from build123d import *

# Parameters (mm, degrees)
SKETCH1_W                          = 55.2
SKETCH1_H                          = 30
SKETCH2_W                          = 90
SKETCH2_H                          = 90
BOSS_EXTRUDE1_DEPTH                = 30
SKETCH8_W                          = 96.2
SKETCH8_H                          = 30
SKETCH11_W                         = 100.2
SKETCH11_H                         = 27
SKETCH15_W                         = 2.5
SKETCH15_H                         = 30
SKETCH16_W                         = 20
SKETCH16_H                         = 71.644187242
CUT_EXTRUDE1_DEPTH                 = 55.2
SKETCH17_OUTSIDE_W                 = 124.71
SKETCH17_OUTSIDE_H                 = 124.71
SKETCH17_OUTSIDE_W_2               = 50
SKETCH17_OUTSIDE_H_2               = 73.870600334
CUT_EXTRUDE2_DEPTH                 = 55.2
SKETCH19_R                         = 10
CUT_EXTRUDE3_DEPTH                 = 133.182790105
CUT_EXTRUDE4_DEPTH                 = 133.182790105
TAP_DRILL_FOR_M1_2X0_25_TAP2_D     = 48
TAP_DRILL_FOR_M1_2X0_25_TAP2_DEPTH = 25
TAP_DRILL_FOR_M1_2X0_25_TAP2_TIP   = 14.420654857
CIRPATTERN1_COUNT                  = 4
M16X1_5_TAPPED_HOLE3_D             = 14.5
M16X1_5_TAPPED_HOLE3_DEPTH         = 16
M16X1_5_TAPPED_HOLE3_TIP           = 4.356239488
CUT_EXTRUDE5_REACH                 = 145.779
SKETCH45_R                         = 1.7


with BuildPart() as part:
    # Sketch1 → Revolve-Thin1 (revolve)
    with BuildSketch(Plane.XY, mode=Mode.PRIVATE) as revolve_thin1_sk:
        with Locations((27.6, 15)):
            Rectangle(SKETCH1_W, SKETCH1_H)
    revolve(revolve_thin1_sk.sketch.rotate(Axis((0, 0, 0), (1, 0, 0)), 90), axis=Axis((0, 0, 0), (1, 0, 0)))

    # Sketch2 → Boss-Extrude1 (add)
    with BuildSketch(Plane(origin=(55.2, 0, 0), x_dir=(0, 0, -1), z_dir=(1, 0, 0))):
        Rectangle(SKETCH2_W, SKETCH2_H)
    extrude(amount=BOSS_EXTRUDE1_DEPTH)

    # Sketch8 → Revolve-Thin2 (revolve)
    with BuildSketch(Plane.XY, mode=Mode.PRIVATE) as revolve_thin2_sk:
        with Locations((48.1, 15)):
            Rectangle(SKETCH8_W, SKETCH8_H)
    revolve(revolve_thin2_sk.sketch.rotate(Axis((0, 0, 0), (1, 0, 0)), 90), axis=Axis((0, 0, 0), (1, 0, 0)))

    # Sketch11 → Revolve-Thin3 (revolve)
    with BuildSketch(Plane(origin=(0, 0, 0), x_dir=(1, 0, 0), z_dir=(0, 1, 0)), mode=Mode.PRIVATE) as revolve_thin3_sk:
        with Locations((50.1, 13.5)):
            Rectangle(SKETCH11_W, SKETCH11_H)
    revolve(revolve_thin3_sk.sketch.rotate(Axis((0, 0, 0), (1, 0, 0)), 180), axis=Axis((0, 0, 0), (1, 0, 0)))

    # Sketch15 → Revolve-Thin4 (revolve)
    with BuildSketch(Plane.XY, mode=Mode.PRIVATE) as revolve_thin4_sk:
        with Locations((101.45, 15)):
            Rectangle(SKETCH15_W, SKETCH15_H)
    revolve(revolve_thin4_sk.sketch.rotate(Axis((100.2, 0, 0), (1, 0, 0)), 90), axis=Axis((100.2, 0, 0), (1, 0, 0)))

    # Sketch16 → Cut-Extrude1 (cut)
    with BuildSketch(Plane.ZY):
        Rectangle(SKETCH16_W, SKETCH16_H)
    extrude(amount=-CUT_EXTRUDE1_DEPTH, mode=Mode.SUBTRACT)

    # Sketch17 outside → Cut-Extrude2 (cut)
    with BuildSketch(Plane.ZY):
        Rectangle(SKETCH17_OUTSIDE_W, SKETCH17_OUTSIDE_H)
        Rectangle(SKETCH17_OUTSIDE_W_2, SKETCH17_OUTSIDE_H_2, mode=Mode.SUBTRACT)
    extrude(amount=-CUT_EXTRUDE2_DEPTH, mode=Mode.SUBTRACT)

    # Sketch19 → Cut-Extrude3 (cut, through all)
    with BuildSketch(Plane.XY.offset(25)):
        with Locations((25.2, 0)):
            Circle(SKETCH19_R)
    extrude(amount=-CUT_EXTRUDE3_DEPTH, mode=Mode.SUBTRACT)

    # Sketch22 → Cut-Extrude4 (cut, through all)
    with BuildSketch(Plane(origin=(0, 0, -25), x_dir=(-1, 0, 0), z_dir=(0, 0, -1))):
        with BuildLine():
            Line((0, 16.583123952), (-5, 16.583123952))
            ThreePointArc((-5, 16.583123952), (-1.277186767, 8.660254038), (0, 0))
            Line((0, 0), (0, 16.583123952))
        make_face()
        with BuildLine():
            Line((9.98487255, 34.360502565), (-23.649851102, 34.360502565))
            Line((-23.649851102, 34.360502565), (-23.649851102, 29.320225254))
            ThreePointArc((-23.649851102, 29.320225254), (-13.080591134, 24.773647362), (-5, 16.583123952))
            Line((-5, 16.583123952), (0, 16.583123952))
            Line((0, 16.583123952), (0, 0))
            Line((0, 0), (0, -16.583123952))
            Line((0, -16.583123952), (-5, -16.583123952))
            ThreePointArc((-5, -16.583123952), (-13.080591134, -24.773647362), (-23.649851102, -29.320225254))
            Line((-23.649851102, -29.320225254), (-23.649851102, -35.668103598))
            Line((-23.649851102, -35.668103598), (9.98487255, -35.668103598))
            Line((9.98487255, -35.668103598), (9.98487255, 34.360502565))
        make_face()
        with BuildLine():
            Line((0, -16.583123952), (0, 0))
            ThreePointArc((0, 0), (-1.277186767, -8.660254038), (-5, -16.583123952))
            Line((-5, -16.583123952), (0, -16.583123952))
        make_face()
    extrude(amount=-CUT_EXTRUDE4_DEPTH, mode=Mode.SUBTRACT)

    # Tap Drill for M1.2x0.25 Tap2
    with Locations(Plane(origin=(102.7, 0, 0), x_dir=(0, 0, -1), z_dir=(1, 0, 0))):
        with Locations((0, 0)):
            Hole(TAP_DRILL_FOR_M1_2X0_25_TAP2_D / 2, depth=TAP_DRILL_FOR_M1_2X0_25_TAP2_DEPTH)
            with Locations((0, 0, -(TAP_DRILL_FOR_M1_2X0_25_TAP2_DEPTH + TAP_DRILL_FOR_M1_2X0_25_TAP2_TIP / 2))):  # 118° drill point
                Cone(0, TAP_DRILL_FOR_M1_2X0_25_TAP2_D / 2, TAP_DRILL_FOR_M1_2X0_25_TAP2_TIP, mode=Mode.SUBTRACT)

    # Sketch32 → M12 Tapped Hole2 (revolve, cut)
    with BuildSketch(Plane(origin=(85.2, -31.819805153, 31.819805153), x_dir=(0, 0, -1), z_dir=(0, 1, 0))):
        Polygon((0, 0), (0, 23.064389157), (5.1, 20), (5.1, 0), align=None)
    m12_tapped_hole2 = revolve(axis=Axis((91.55, -31.819805153, 31.819805153), (-1, 0, 0)), mode=Mode.SUBTRACT)

    # CirPattern1: M12 Tapped Hole2 ×4 about axis
    cirpattern1_axis = Axis((0, 0, 0), (1, 0, 0))
    for i in range(1, CIRPATTERN1_COUNT):
        add(m12_tapped_hole2.rotate(cirpattern1_axis, i * 360 / CIRPATTERN1_COUNT), mode=Mode.SUBTRACT)

    # M16x1.5 Tapped Hole3
    with Locations(Plane(origin=(70.2, -45, 0), x_dir=(0, 0, -1), z_dir=(0, -1, 0))):
        with Locations((0, 0)):
            Hole(M16X1_5_TAPPED_HOLE3_D / 2, depth=M16X1_5_TAPPED_HOLE3_DEPTH)
            with Locations((0, 0, -(M16X1_5_TAPPED_HOLE3_DEPTH + M16X1_5_TAPPED_HOLE3_TIP / 2))):  # 118° drill point
                Cone(0, M16X1_5_TAPPED_HOLE3_D / 2, M16X1_5_TAPPED_HOLE3_TIP, mode=Mode.SUBTRACT)

    # Cut-Extrude5: up to this cone (the profile starts outside it)
    cut_extrude5_end = Plane(origin=(70.2, 0, 0), z_dir=(1, 0, 0)).offset(-6.920653857) * Cone(1.664e-06, 274.136053392, 164.717557739, align=(Align.CENTER, Align.CENTER, Align.MIN), mode=Mode.PRIVATE)
    # Sketch45 → Cut-Extrude5 (cut, up to the surface)
    with BuildSketch(Plane.XZ.offset(45), mode=Mode.PRIVATE) as cut_extrude5_sk1:
        with Locations(Location((70.2, 0, 0), (0, 0, 270))):
            Circle(SKETCH45_R)
    cut_extrude5_tool1 = extrude(cut_extrude5_sk1.sketch, amount=-CUT_EXTRUDE5_REACH, mode=Mode.PRIVATE) - cut_extrude5_end
    add(cut_extrude5_tool1.solids().sort_by_distance((70.2, -45, 0))[0], mode=Mode.SUBTRACT)


solid = part.part
Read the model definition and answer for the solid it produces. Units are mm, in the model's axes. A direction names the side the tool comes from. Give positions to 0.01 mm unless a question says otherwise; leave off trailing zeros. Loops run counter-clockwise (first coordinate to the right, second up) from the corner with the lowest first, then second, coordinate; pieces in that order, holes last. Notation, with made-up numbers: (45, 64.5) - (86, 64.5) arc R29 cw to (86, 96.5) - close; hole circle Ø8 at (-7, 64.5). An arc over 180 degrees is marked (long way). Answer as CSV lines item,"result". Start each with the question number.
1) Find section B-B (x = 93). Write down the section's boundary in (y, z), then the cut area to 3 significant figures.
2) Determine the mould class of faces 1 (the face through (62.67, 31.03, -31.41)), 2 (the face through (75.34, -29.866, 27.109)), 3 (the face through (98.23, 26.36, -5.85)) for opening direction X: released by +X, released by -X, zero draft, split by the parting line, or undercut.
3) Which of the six approach directions +Z, -Z, +X, -X, +Y, -Y give full straight-line access (tool end or side, diameter ignored) to faces 4 (the face through (101.468, -25.296, 16.128)), 5 (the face through (33, -7, -10)), 6 (the face through (100.2, -11, 25)), 7 (the face through (36, 24, 18))?
4) Find section C-C (x = 70.2). Write down the section's boundary in (y, z).
5) Straight lines are drawn through the part: L1, parallel to Z at x = 14.5, y = -10; L2, parallel to Z at x = 17, y = -18; L3, parallel to Y at x = 77, z = 35. For each, find the intervals that lie inside material, in ascending order. Write a range as from..to.
6) Each of these flat-tipped pins is pushed along its axis until it touches: pin 1 Ø16 at (x, y) = (25.2, 0) entering from -Z; pin 2 Ø8 at (y, z) = (31.82, -31.82) entering from +X; pin 3 Ø6 at (y, z) = (-31.82, 31.82) entering from +X; pin 4 Ø1 at (y, z) = (26.5, -35.5) entering from +X. Where does it stop, or does it pass through?
7) Find section A-A (x = 46). Write down the section's boundary in (y, z), then the cut area to 3 significant figures.
Findings below:
1,outline,"circle Ø60 at (0, 0); hole circle Ø48 at (0, 0)"
1,area,"1,020 mm^2"
2,face 1,"released by +X"
2,face 2,"zero draft"
2,face 3,"undercut"
3,face 4,"+X"
3,face 5,"-X, +Y, -Y"
3,face 6,"none"
3,face 7,"+Z, -X, +Y"
4,outline,"(-45, -45) - (45, -45) - (45, 45) - (-45, 45) - (-45, 7.25) - (-29, 7.25) - (-25.67, 1.7) - (-11.39, 1.7) arc R11.52 cw (long way) to (-11.39, -1.7) - (-25.67, -1.7) - (-29, -7.25) - (-45, -7.25) - close; hole circle Ø10.2 at (-31.82, -31.82); hole circle Ø10.2 at (-31.82, 31.82); hole circle Ø10.2 at (31.82, -31.82); hole circle Ø10.2 at (31.82, 31.82)"
5,L1,"-25..-10, 10..25"
5,L2,"-24..-10, 10..24"
5,L3,"-45..-35.81, -27.83..27.83, 35.81..45"
6,pin 1,"through"
6,pin 2,"x = 64.54"
6,pin 3,"x = 63.94"
6,pin 4,"x = 85.2"
7,outline,"(-28.28, -10) arc R30 ccw to (-16.58, -25) - (16.58, -25) arc R30 ccw to (28.28, -10) - close; (-28.28, 10) - (28.28, 10) arc R30 ccw to (16.58, 25) - (-16.58, 25) arc R30 ccw to start"
7,area,"1,420 mm^2"
